Geometry: final body of the model. Coordinates: model frame, mm. A direction names the side the tool comes from. Give positions to 0.01 mm unless a question says otherwise; leave off trailing zeros. Loops run counter-clockwise (first coordinate to the right, second up) from the corner with the lowest first, then second, coordinate; pieces in that order, holes last. Notation, with made-up numbers: (82.25, -38.5) -> (102.25, -38.5) arc R28 ccw to (102.25, -18.5) -> close; hole circle Ø5 at (17, 31). An arc over 180 degrees is marked (long way). Answer in a Markdown table with one row per item. Add a question column.
1) Access query for faces 1 (the flat face through (0, 19.05, -1)), 2 (the flat face through (-9, 9, 15.24)), 3 (the cylindrical face through (-11.172, 9.658, -23.951)). Directions: +Z, -Z, +X, -X, +Y, -Y. A direction counts if a zero-diameter tool reaches every point of the face in a straight line with its end or side. Return the directions, or none.
2) Line query: line 1 (Z direction, x = -3.5, y = 17); line 2 (Y direction, x = 0, z = 30.25); line 3 (Z direction, x = -22, y = 16.75). Output: solid intervals per line, ascending. Write a range as from..to.
3) Section query B-B (x = -14). Return the cut outline in (y, z).
4) First-contact query: P1, Ø10, axis at x = 0, y = 9.525, coming from the +Z side; P2, Ø10, axis at x = -16.5, z = 22, coming from the +Y side. Flat tips, straight axial feed; report the tip coordinate or a pass-through.
5) Section query A-A (x = 0). Return the cut outline in (y, z), plus the area to 3 significant figures.
6) Draft query along Y for faces 4 (the flat face through (25.4, 9, 12)), 5 (the flat face through (0, 0, -1)), 6 (the cylindrical face through (-1.2, 4.1, 31.8)), 7 (the cylindrical face through (-1.2, 4.1, -31.8)). Return one class per face: +Y half, -Y half, draft (parallel to the pull), parting line (faces both ways), or undercut.
7) Section query C-C (y = 4.75). Give the number of separate pieces and of enclosed holes in the cut face, plus the area to 3 significant figures.
```python
from build123d import *

# Parameters (mm, degrees)
BOSS_EXTRUDE1_DEPTH = 19.05
FILLET1_R           = 5.08
CUT_EXTRUDE1_REACH  = 84.55
SKETCH2_R           = 5.55625
CUT_EXTRUDE2_START  = -76.2
SKETCH2_2_R         = 5.55625
CUT_EXTRUDE2_DEPTH  = 12.7


with BuildPart() as part:
    # Sketch1 → Boss-Extrude1 (new body)
    with BuildSketch(Plane(origin=(0, 0, 0), x_dir=(1, 0, 0), z_dir=(0, 1, 0))):
        Polygon((-12.7, 25.4), (25.4, 25.4), (25.4, 38.1), (-25.4, 38.1), (-25.4, -15.24), (12.7, -15.24), (12.7, -25.4), (-25.4, -25.4), (-25.4, -38.1), (25.4, -38.1), (25.4, 15.24), (-12.7, 15.24), align=None)
    extrude(amount=BOSS_EXTRUDE1_DEPTH)

    # Fillet1
    fillet1_edges = [part.edges().sort_by_distance(p)[0] for p in [
        (12.7, 9.525, 25.4),
        (12.7, 9.525, 15.24),
        (-12.7, 9.525, -15.24),
        (-12.7, 9.525, -25.4),
    ]]
    fillet(fillet1_edges, radius=FILLET1_R - 0.0001)  # a hair under: the kernel refuses the full size

    # Sketch2 → Cut-Extrude1 (cut, up to next)
    with BuildSketch(Plane.XY.offset(38.1), mode=Mode.PRIVATE) as cut_extrude1_sk1:
        with Locations((0, 9.525)):
            Circle(SKETCH2_R)
    cut_extrude1_tool1 = extrude(cut_extrude1_sk1.sketch, amount=-CUT_EXTRUDE1_REACH, mode=Mode.PRIVATE) & part.part
    add(cut_extrude1_tool1.solids().sort_by_distance((0, 9.525, 38.1))[0], mode=Mode.SUBTRACT)

    # Sketch2<2> → Cut-Extrude2 (cut)
    with BuildSketch(Plane.XY.offset(38.1).offset(CUT_EXTRUDE2_START)):
        with Locations((0, 9.525)):
            Circle(SKETCH2_2_R)
    extrude(amount=CUT_EXTRUDE2_DEPTH, mode=Mode.SUBTRACT)


solid = part.part
```
Evaluation:
| question | item | result |
|---|---|---|
| 1 | face 1 | +Z, -Z, +X, -X, +Y |
| 1 | face 2 | -X, +Y, -Y |
| 1 | face 3 | +X, +Y, -Y |
| 2 | line 1 | -38.1..-25.4, -15.24..15.24, 25.4..38.1 |
| 2 | line 2 | 0..3.97, 15.08..19.05 |
| 2 | line 3 | -38.1..15.24, 25.4..38.1 |
| 3 | outline | (0, -38.1) -> (19.05, -38.1) -> (19.05, 15.24) -> (0, 15.24) -> close; (0, 25.4) -> (19.05, 25.4) -> (19.05, 38.1) -> (0, 38.1) -> close |
| 4 | P1 | z = 15.24 |
| 4 | P2 | y = 19.05 |
| 5 | outline | (0, -38.1) -> (3.97, -38.1) -> (3.97, -25.4) -> (0, -25.4) -> close; (0, -15.24) -> (19.05, -15.24) -> (19.05, 15.24) -> (0, 15.24) -> close; (0, 25.4) -> (3.97, 25.4) -> (3.97, 38.1) -> (0, 38.1) -> close; (15.08, -38.1) -> (19.05, -38.1) -> (19.05, -25.4) -> (15.08, -25.4) -> close; (15.08, 25.4) -> (19.05, 25.4) -> (19.05, 38.1) -> (15.08, 38.1) -> close |
| 5 | area | 782 mm² |
| 6 | face 4 | draft |
| 6 | face 5 | -Y half |
| 6 | face 6 | undercut |
| 6 | face 7 | undercut |
| 7 | separate pieces | 3 |
| 7 | enclosed holes | 0 |
| 7 | area | 2,970 mm² |
